Geometry check sheet. Reference: the model listing, model coordinates, mm. Coordinates: 2 decimals unless noted, no trailing zeros. Loops run counter-clockwise (first coordinate to the right, second up) from the corner with the lowest first, then second, coordinate; pieces in that order, holes last. Notation, with made-up numbers: M 70.25,47.25 L 116.25,47.25 A19 cw 116.25,77.25 Z; hole C -32,-4 d3. An arc over 180 degrees is marked long. One line per question, with ' | ' between items. Start each with the question number.
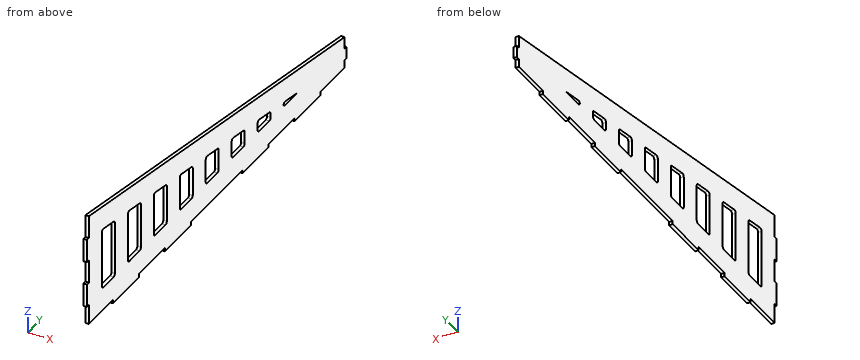
from build123d import *

# Parameters (mm, degrees)
BOSS_EXTRUDE1_DEPTH = 3
SKETCH2_W           = 20
SKETCH2_H           = 3
SKETCH2_W_2         = 3
SKETCH2_H_2         = 40
SKETCH2_H_3         = 80
CUT_EXTRUDE1_DEPTH  = 3
CUT_EXTRUDE2_DEPTH  = 3
FILLET1_R           = 2


with BuildPart() as part:
    # Sketch1 → Boss-Extrude1 (new body)
    with BuildSketch(Plane(origin=(0, 0, 0), x_dir=(0, 0, -1), z_dir=(1, 0, 0))):
        Polygon((0, 183.89261745), (0, -216.10738255), (-100, -216.10738255), (-30, 183.89261745), align=None)
    extrude(amount=BOSS_EXTRUDE1_DEPTH)

    # Sketch2 → Cut-Extrude1 (cut)
    with BuildSketch(Plane(origin=(3, 0, 0), x_dir=(0, 0, -1), z_dir=(1, 0, 0))):
        Polygon((-80, -213.10738255), (-99.475, -213.10738255), (-100, -216.10738255), (-80, -216.10738255), align=None)
        Polygon((-30, 183.89261745), (-30.525, 180.89261745), (-20, 180.89261745), (-20, 183.89261745), align=None)
        with Locations((-50, -214.60738255)):
            Rectangle(SKETCH2_W, SKETCH2_H)
        Polygon((-3, -213.10738255), (-20, -213.10738255), (-20, -216.10738255), (0, -216.10738255), (0, -176.10738255), (-3, -176.10738255), align=None)
        Polygon((-10, 183.89261745), (-10, 180.89261745), (-3, 180.89261745), (-3, 143.89261745), (0, 143.89261745), (0, 183.89261745), align=None)
        with Locations((-1.5, -116.10738255)):
            Rectangle(SKETCH2_W_2, SKETCH2_H_2)
        with Locations((-1.5, 83.89261745)):
            Rectangle(SKETCH2_W_2, SKETCH2_H_2)
        with Locations((-1.5, -16.10738255)):
            Rectangle(SKETCH2_W_2, SKETCH2_H_3)
    extrude(amount=-CUT_EXTRUDE1_DEPTH, mode=Mode.SUBTRACT)

    # Sketch3 → Cut-Extrude2 (cut)
    with BuildSketch(Plane(origin=(3, 0, 0), x_dir=(0, 0, -1), z_dir=(1, 0, 0))):
        Polygon((-68.671059496, -153.10738255), (-65.171059496, -133.10738255), (-23, -133.10738255), (-23, -153.10738255), align=None)
        Polygon((-23, -173.10738255), (-23, -193.10738255), (-75.671059496, -193.10738255), (-72.171059496, -173.10738255), align=None)
        Polygon((-61.671059496, -113.10738255), (-58.171059496, -93.10738255), (-23, -93.10738255), (-23, -113.10738255), align=None)
        Polygon((-54.671059496, -73.10738255), (-51.171059496, -53.10738255), (-23, -53.10738255), (-23, -73.10738255), align=None)
        Polygon((-23, 107.870100283), (-23, 86.89261745), (-26.671059496, 86.89261745), align=None)
        Polygon((-23, -33.10738255), (-47.671059496, -33.10738255), (-44.171059496, -13.10738255), (-23, -13.10738255), align=None)
        Polygon((-23, 6.89261745), (-40.671059496, 6.89261745), (-37.171059496, 26.89261745), (-23, 26.89261745), align=None)
        Polygon((-23, 46.89261745), (-33.671059496, 46.89261745), (-30.171059496, 66.89261745), (-23, 66.89261745), align=None)
    extrude(amount=-CUT_EXTRUDE2_DEPTH, mode=Mode.SUBTRACT)

    # Fillet1
    # the kernel refuses this fillet: 2 mm, written as the material it adds along each edge
    with BuildSketch(Plane(origin=(3, 86.89261745, 26.671059496), x_dir=(0, 0, -1), z_dir=(-1, 0, 0)), Plane(origin=(3, 46.89261745, 33.671059496), x_dir=(0, 0, -1), z_dir=(-1, 0, 0)), Plane(origin=(3, 6.89261745, 40.671059496), x_dir=(0, 0, -1), z_dir=(-1, 0, 0)), Plane(origin=(3, -33.10738255, 47.671059496), x_dir=(0, 0, -1), z_dir=(-1, 0, 0)), Plane(origin=(3, -193.10738255, 75.671059496), x_dir=(0, 0, -1), z_dir=(-1, 0, 0))) as fillet1_piece_1:
        with BuildLine():
            CenterArc((FILLET1_R * 1.19019702521, -FILLET1_R), FILLET1_R, 90, 99.926245507)
            Line((FILLET1_R * 0.205166558057, -FILLET1_R * 1.17238033175), (0, 0))
            Line((0, 0), (FILLET1_R * 1.19019702521, 0))
        make_face()
    extrude(amount=3)
    with BuildSketch(Plane(origin=(3, 86.89261745, 23), x_dir=(0, 1, 0), z_dir=(-1, 0, 0)), Plane(origin=(3, 66.89261745, 23), x_dir=(0, 0, 1), z_dir=(-1, 0, 0)), Plane(origin=(3, 26.89261745, 23), x_dir=(0, 0, 1), z_dir=(-1, 0, 0)), Plane(origin=(3, -13.10738255, 23), x_dir=(0, 0, 1), z_dir=(-1, 0, 0)), Plane(origin=(3, -93.10738255, 23), x_dir=(0, 0, 1), z_dir=(-1, 0, 0)), Plane(origin=(3, -73.10738255, 23), x_dir=(0, 1, 0), z_dir=(-1, 0, 0)), Plane(origin=(3, -53.10738255, 23), x_dir=(0, 0, 1), z_dir=(-1, 0, 0)), Plane(origin=(3, -133.10738255, 23), x_dir=(0, 0, 1), z_dir=(-1, 0, 0)), Plane(origin=(3, -113.10738255, 23), x_dir=(0, 1, 0), z_dir=(-1, 0, 0)), Plane(origin=(3, -153.10738255, 23), x_dir=(0, 1, 0), z_dir=(-1, 0, 0)), Plane(origin=(3, -193.10738255, 23), x_dir=(0, 1, 0), z_dir=(-1, 0, 0))) as fillet1_piece_2:
        with BuildLine():
            CenterArc((FILLET1_R, -FILLET1_R), FILLET1_R, 90, 90)
            Line((0, -FILLET1_R), (0, 0))
            Line((0, 0), (FILLET1_R, 0))
        make_face()
    extrude(amount=3)
    with BuildSketch(Plane(origin=(3, 66.89261745, 30.171059496), x_dir=(0, -0.985030467155704, 0.17238033175224968), z_dir=(-1, 0, 0)), Plane(origin=(3, 26.89261745, 37.171059496), x_dir=(0, -0.9850304671557044, 0.172380331752247), z_dir=(-1, 0, 0)), Plane(origin=(3, -13.10738255, 44.171059496), x_dir=(0, -0.9850304671557039, 0.1723803317522504), z_dir=(-1, 0, 0)), Plane(origin=(3, -53.10738255, 51.171059496), x_dir=(0, -0.9850304671557039, 0.1723803317522504), z_dir=(-1, 0, 0)), Plane(origin=(3, -93.10738255, 58.171059496), x_dir=(0, -0.9850304671557047, 0.17238033175224557), z_dir=(-1, 0, 0)), Plane(origin=(3, -133.10738255, 65.171059496), x_dir=(0, -0.9850304671557039, 0.17238033175224987), z_dir=(-1, 0, 0)), Plane(origin=(3, -173.10738255, 72.171059496), x_dir=(0, -0.9850304671557039, 0.17238033175224987), z_dir=(-1, 0, 0))) as fillet1_piece_3:
        with BuildLine():
            CenterArc((FILLET1_R * 0.840197025212, -FILLET1_R), FILLET1_R, 90, 80.073754493)
            Line((-FILLET1_R * 0.144833441943, -FILLET1_R * 0.827619668248), (0, 0))
            Line((0, 0), (FILLET1_R * 0.840197025212, 0))
        make_face()
    extrude(amount=3)
    with BuildSketch(Plane(origin=(3, 46.89261745, 23), x_dir=(0, 0, 1), z_dir=(-1, 0, 0)), Plane(origin=(3, 6.89261745, 23), x_dir=(0, 0, 1), z_dir=(-1, 0, 0)), Plane(origin=(3, -33.10738255, 23), x_dir=(0, 0, 1), z_dir=(-1, 0, 0)), Plane(origin=(3, -173.10738255, 23), x_dir=(0, -1, 0), z_dir=(-1, 0, 0))) as fillet1_piece_4:
        with BuildLine():
            CenterArc((FILLET1_R, FILLET1_R), FILLET1_R, 180, 90)
            Line((0, FILLET1_R), (0, 0))
            Line((0, 0), (FILLET1_R, 0))
        make_face()
    extrude(amount=3)
    with BuildSketch(Plane(origin=(3, -73.10738255, 54.671059496), x_dir=(0, 0.985030467155704, -0.17238033175224923), z_dir=(-1, 0, 0)), Plane(origin=(3, -113.10738255, 61.671059496), x_dir=(0, 0.9850304671557042, -0.17238033175224837), z_dir=(-1, 0, 0)), Plane(origin=(3, -153.10738255, 68.671059496), x_dir=(0, 0.9850304671557039, -0.17238033175225026), z_dir=(-1, 0, 0))) as fillet1_piece_5:
        with BuildLine():
            CenterArc((FILLET1_R * 1.19019702521, FILLET1_R), FILLET1_R, 170.073754493, 99.926245507)
            Line((FILLET1_R * 0.205166558057, FILLET1_R * 1.17238033175), (0, 0))
            Line((0, 0), (FILLET1_R * 1.19019702521, 0))
        make_face()
    extrude(amount=3)


solid = part.part
1. Depth check by flat-ended pin: pin 1 Ø1 at (x, y) = (1.5, 57.5) entering from +Z. Enter the tip coordinate at first touch or a pass-through.
2. Thickness scan on line 1 (Z direction, x = 0.35, y = -18); line 2 (Y direction, x = 0.2, z = 18); line 3 (Z direction, x = 2.3, y = 104). Record the ranges inside material, lowest first.
3. Sectioned sample at B-B (x = 1.85). State how many separate pieces and enclosed holes the cut face has, and give its area (3 significant figures).
4. Sectioned sample at A-A (y = -20.5). Record the cut outline in (x, z).
5. Sectioned sample at C-C (z = 87). Record the cut outline in (x, y), and give its area (3 significant figures).
6. Sectioned sample at D-D (y = 152). Record the cut outline in (x, z), and give its area (3 significant figures).
Result:
1) pin 1: stops at z = 52.21
2) line 1: z = 3 to 23, 45.03 to 65.33 | line 2: y = -213.11 to 183.89 | line 3: z = 0 to 23, 23.68 to 43.98
3) separate pieces: 1 | enclosed holes: 8 | area: 20,900 mm2
4) outline: M 0,3 L 3,3 L 3,23 L 0,23 Z; M 0,45.46 L 3,45.46 L 3,65.77 L 0,65.77 Z
5) outline: M 0,-213.11 L 3,-213.11 L 3,-141.82 L 0,-141.82 Z | area: 214 mm2
6) outline: M 0,3 L 3,3 L 3,35.58 L 0,35.58 Z | area: 97.7 mm2
